```python
from build123d import *

# Parameters (mm, degrees)
BASE_SKETCH_W              = 127
BASE_SKETCH_H              = 147.5
BASE_SKETCH_R              = 5
BASE_DEPTH                 = 3
LEGS_SKETCH_W              = 5
LEGS_SKETCH_H              = 15
LEGS_DEPTH                 = 5
MOUNT_SKETCH_W             = 15
MOUNT_SKETCH_H             = 1
MOUNT_DEPTH                = 6
DONT_CUT_URSELF_R          = 6
MOUNTING_HOLE_SKETCH_R     = 1.5
MOUNTING_HOLE_1_DEPTH      = 2
MOUNTING_HOLE_2_SKETCH_R   = 1.5
MOUNTING_HOLE_2_DEPTH      = 2
MOUNT_2_SKETCH_W           = 15
MOUNT_2_SKETCH_H           = 1
MOUNT_2_DEPTH              = 6
DONT_CUT_URSELF_2_R        = 6
MOUNTING_HOLE_3_SKETCH_R   = 1.5
MOUNTING_HOLE_3_DEPTH      = 2
MOUNTING_HOLE_4_SKETCH_R   = 1.5
MOUNTING_HOLE_4_DEPTH      = 2
HOLES_FOR_PARTS_REACH      = 10
HOLES_FOR_PARTS_SKETCH_R   = 1.5
HOLES_FOR_PARTS_SKETCH_R_2 = 1.59


with BuildPart() as part:
    # Base Sketch → Base (new body)
    with BuildSketch(Plane(origin=(0, 0, 0), x_dir=(1, 0, 0), z_dir=(0, 1, 0))):
        Rectangle(BASE_SKETCH_W, BASE_SKETCH_H)
        Circle(BASE_SKETCH_R, mode=Mode.SUBTRACT)
    extrude(amount=BASE_DEPTH)

    # Legs Sketch → Legs (add)
    with BuildSketch(Plane.XZ):
        with Locations((-61, -66.25)):
            Rectangle(LEGS_SKETCH_W, LEGS_SKETCH_H)
        with Locations((61, -66.25)):
            Rectangle(LEGS_SKETCH_W, LEGS_SKETCH_H)
        with Locations((-61, 66.25)):
            Rectangle(LEGS_SKETCH_W, LEGS_SKETCH_H)
        with Locations((61, 66.25)):
            Rectangle(LEGS_SKETCH_W, LEGS_SKETCH_H)
    extrude(amount=LEGS_DEPTH)

    # Mount Sketch → Mount (add)
    with BuildSketch(Plane(origin=(63.5, 0, 0), x_dir=(0, 0, -1), z_dir=(1, 0, 0))):
        with Locations((-66.25, -4.5)):
            Rectangle(MOUNT_SKETCH_W, MOUNT_SKETCH_H)
        with Locations((66.25, -4.5)):
            Rectangle(MOUNT_SKETCH_W, MOUNT_SKETCH_H)
    extrude(amount=MOUNT_DEPTH)

    # Dont cut urself
    dont_cut_urself_edges = [part.edges().sort_by_distance(p)[0] for p in [
        (69.5, -4.5, 58.75),
        (69.5, -4.5, 73.75),
        (69.5, -4.5, -73.75),
        (69.5, -4.5, -58.75),
    ]]
    fillet(dont_cut_urself_edges, radius=DONT_CUT_URSELF_R)

    # Mounting Hole Sketch → Mounting Hole 1 (cut, through all)
    with BuildSketch(Plane(origin=(0, -4, 0), x_dir=(1, 0, 0), z_dir=(0, 1, 0))):
        with Locations((66.5, -66.25)):
            Circle(MOUNTING_HOLE_SKETCH_R)
    extrude(amount=-MOUNTING_HOLE_1_DEPTH, mode=Mode.SUBTRACT)

    # Mounting Hole 2 Sketch → Mounting Hole 2 (cut, through all)
    with BuildSketch(Plane(origin=(0, -4, 0), x_dir=(1, 0, 0), z_dir=(0, 1, 0))):
        with Locations((66.5, 66.25)):
            Circle(MOUNTING_HOLE_2_SKETCH_R)
    extrude(amount=-MOUNTING_HOLE_2_DEPTH, mode=Mode.SUBTRACT)

    # Mount 2 Sketch → Mount 2 (add)
    with BuildSketch(Plane.ZY.offset(63.5)):
        with Locations((-66.25, -4.5)):
            Rectangle(MOUNT_2_SKETCH_W, MOUNT_2_SKETCH_H)
        with Locations((66.25, -4.5)):
            Rectangle(MOUNT_2_SKETCH_W, MOUNT_2_SKETCH_H)
    extrude(amount=MOUNT_2_DEPTH)

    # Dont cut urself 2
    dont_cut_urself_2_edges = [part.edges().sort_by_distance(p)[0] for p in [
        (-69.5, -4.5, 73.75),
        (-69.5, -4.5, 58.75),
        (-69.5, -4.5, -58.75),
        (-69.5, -4.5, -73.75),
    ]]
    fillet(dont_cut_urself_2_edges, radius=DONT_CUT_URSELF_2_R)

    # Mounting Hole 3 Sketch → Mounting Hole 3 (cut, through all)
    with BuildSketch(Plane(origin=(0, -4, 0), x_dir=(1, 0, 0), z_dir=(0, 1, 0))):
        with Locations((-66.5, -66.25)):
            Circle(MOUNTING_HOLE_3_SKETCH_R)
    extrude(amount=-MOUNTING_HOLE_3_DEPTH, mode=Mode.SUBTRACT)

    # Mounting Hole 4 Sketch → Mounting Hole 4 (cut, through all)
    with BuildSketch(Plane(origin=(0, -4, 0), x_dir=(1, 0, 0), z_dir=(0, 1, 0))):
        with Locations((-66.5, 66.25)):
            Circle(MOUNTING_HOLE_4_SKETCH_R)
    extrude(amount=-MOUNTING_HOLE_4_DEPTH, mode=Mode.SUBTRACT)

    # Holes for Parts Sketch → Holes for Parts (cut, up to next)
    with BuildSketch(Plane(origin=(0, 3, 0), x_dir=(1, 0, 0), z_dir=(0, 1, 0)), mode=Mode.PRIVATE) as holes_for_parts_sk1:
        with Locations((31.75, -68.75)):
            Circle(HOLES_FOR_PARTS_SKETCH_R)
    holes_for_parts_tool1 = extrude(holes_for_parts_sk1.sketch, amount=-HOLES_FOR_PARTS_REACH, mode=Mode.PRIVATE) & part.part
    add(holes_for_parts_tool1.solids().sort_by_distance((31.75, 3, 68.75))[0], mode=Mode.SUBTRACT)
    # Holes for Parts Sketch → Holes for Parts (cut, up to next)
    with BuildSketch(Plane(origin=(0, 3, 0), x_dir=(1, 0, 0), z_dir=(0, 1, 0)), mode=Mode.PRIVATE) as holes_for_parts_sk2:
        with Locations((58.5, -53.875)):
            Circle(HOLES_FOR_PARTS_SKETCH_R)
    holes_for_parts_tool2 = extrude(holes_for_parts_sk2.sketch, amount=-HOLES_FOR_PARTS_REACH, mode=Mode.PRIVATE) & part.part
    add(holes_for_parts_tool2.solids().sort_by_distance((58.5, 3, 53.875))[0], mode=Mode.SUBTRACT)
    # Holes for Parts Sketch → Holes for Parts (cut, up to next)
    with BuildSketch(Plane(origin=(0, 3, 0), x_dir=(1, 0, 0), z_dir=(0, 1, 0)), mode=Mode.PRIVATE) as holes_for_parts_sk3:
        with Locations((5, -53.875)):
            Circle(HOLES_FOR_PARTS_SKETCH_R)
    holes_for_parts_tool3 = extrude(holes_for_parts_sk3.sketch, amount=-HOLES_FOR_PARTS_REACH, mode=Mode.PRIVATE) & part.part
    add(holes_for_parts_tool3.solids().sort_by_distance((5, 3, 53.875))[0], mode=Mode.SUBTRACT)
    # Holes for Parts Sketch → Holes for Parts (cut, up to next)
    with BuildSketch(Plane(origin=(0, 3, 0), x_dir=(1, 0, 0), z_dir=(0, 1, 0)), mode=Mode.PRIVATE) as holes_for_parts_sk4:
        with Locations((19.75, -15.25)):
            Circle(HOLES_FOR_PARTS_SKETCH_R)
    holes_for_parts_tool4 = extrude(holes_for_parts_sk4.sketch, amount=-HOLES_FOR_PARTS_REACH, mode=Mode.PRIVATE) & part.part
    add(holes_for_parts_tool4.solids().sort_by_distance((19.75, 3, 15.25))[0], mode=Mode.SUBTRACT)
    # Holes for Parts Sketch → Holes for Parts (cut, up to next)
    with BuildSketch(Plane(origin=(0, 3, 0), x_dir=(1, 0, 0), z_dir=(0, 1, 0)), mode=Mode.PRIVATE) as holes_for_parts_sk5:
        with Locations((-50.5, -16.25)):
            Circle(HOLES_FOR_PARTS_SKETCH_R)
    holes_for_parts_tool5 = extrude(holes_for_parts_sk5.sketch, amount=-HOLES_FOR_PARTS_REACH, mode=Mode.PRIVATE) & part.part
    add(holes_for_parts_tool5.solids().sort_by_distance((-50.5, 3, 16.25))[0], mode=Mode.SUBTRACT)
    # Holes for Parts Sketch → Holes for Parts (cut, up to next)
    with BuildSketch(Plane(origin=(0, 3, 0), x_dir=(1, 0, 0), z_dir=(0, 1, 0)), mode=Mode.PRIVATE) as holes_for_parts_sk6:
        with Locations((-24.5, -16.25)):
            Circle(HOLES_FOR_PARTS_SKETCH_R)
    holes_for_parts_tool6 = extrude(holes_for_parts_sk6.sketch, amount=-HOLES_FOR_PARTS_REACH, mode=Mode.PRIVATE) & part.part
    add(holes_for_parts_tool6.solids().sort_by_distance((-24.5, 3, 16.25))[0], mode=Mode.SUBTRACT)
    # Holes for Parts Sketch → Holes for Parts (cut, up to next)
    with BuildSketch(Plane(origin=(0, 3, 0), x_dir=(1, 0, 0), z_dir=(0, 1, 0)), mode=Mode.PRIVATE) as holes_for_parts_sk7:
        with Locations((-7.54, 33.19)):
            Circle(HOLES_FOR_PARTS_SKETCH_R_2)
    holes_for_parts_tool7 = extrude(holes_for_parts_sk7.sketch, amount=-HOLES_FOR_PARTS_REACH, mode=Mode.PRIVATE) & part.part
    add(holes_for_parts_tool7.solids().sort_by_distance((-7.54, 3, -33.19))[0], mode=Mode.SUBTRACT)
    # Holes for Parts Sketch → Holes for Parts (cut, up to next)
    with BuildSketch(Plane(origin=(0, 3, 0), x_dir=(1, 0, 0), z_dir=(0, 1, 0)), mode=Mode.PRIVATE) as holes_for_parts_sk8:
        with Locations((-7.54, 61.13)):
            Circle(HOLES_FOR_PARTS_SKETCH_R_2)
    holes_for_parts_tool8 = extrude(holes_for_parts_sk8.sketch, amount=-HOLES_FOR_PARTS_REACH, mode=Mode.PRIVATE) & part.part
    add(holes_for_parts_tool8.solids().sort_by_distance((-7.54, 3, -61.13))[0], mode=Mode.SUBTRACT)
    # Holes for Parts Sketch → Holes for Parts (cut, up to next)
    with BuildSketch(Plane(origin=(0, 3, 0), x_dir=(1, 0, 0), z_dir=(0, 1, 0)), mode=Mode.PRIVATE) as holes_for_parts_sk9:
        with Locations((44.53, 66.21)):
            Circle(HOLES_FOR_PARTS_SKETCH_R_2)
    holes_for_parts_tool9 = extrude(holes_for_parts_sk9.sketch, amount=-HOLES_FOR_PARTS_REACH, mode=Mode.PRIVATE) & part.part
    add(holes_for_parts_tool9.solids().sort_by_distance((44.53, 3, -66.21))[0], mode=Mode.SUBTRACT)
    # Holes for Parts Sketch → Holes for Parts (cut, up to next)
    with BuildSketch(Plane(origin=(0, 3, 0), x_dir=(1, 0, 0), z_dir=(0, 1, 0)), mode=Mode.PRIVATE) as holes_for_parts_sk10:
        with Locations((43.26, 17.95)):
            Circle(HOLES_FOR_PARTS_SKETCH_R_2)
    holes_for_parts_tool10 = extrude(holes_for_parts_sk10.sketch, amount=-HOLES_FOR_PARTS_REACH, mode=Mode.PRIVATE) & part.part
    add(holes_for_parts_tool10.solids().sort_by_distance((43.26, 3, -17.95))[0], mode=Mode.SUBTRACT)
    # Holes for Parts Sketch → Holes for Parts (cut, up to next)
    with BuildSketch(Plane(origin=(0, 3, 0), x_dir=(1, 0, 0), z_dir=(0, 1, 0)), mode=Mode.PRIVATE) as holes_for_parts_sk11:
        with Locations((50.5, -60.75)):
            Circle(HOLES_FOR_PARTS_SKETCH_R)
    holes_for_parts_tool11 = extrude(holes_for_parts_sk11.sketch, amount=-HOLES_FOR_PARTS_REACH, mode=Mode.PRIVATE) & part.part
    add(holes_for_parts_tool11.solids().sort_by_distance((50.5, 3, 60.75))[0], mode=Mode.SUBTRACT)
    # Holes for Parts Sketch → Holes for Parts (cut, up to next)
    with BuildSketch(Plane(origin=(0, 3, 0), x_dir=(1, 0, 0), z_dir=(0, 1, 0)), mode=Mode.PRIVATE) as holes_for_parts_sk12:
        with Locations((13, -60.75)):
            Circle(HOLES_FOR_PARTS_SKETCH_R)
    holes_for_parts_tool12 = extrude(holes_for_parts_sk12.sketch, amount=-HOLES_FOR_PARTS_REACH, mode=Mode.PRIVATE) & part.part
    add(holes_for_parts_tool12.solids().sort_by_distance((13, 3, 60.75))[0], mode=Mode.SUBTRACT)
    # Holes for Parts Sketch → Holes for Parts (cut, up to next)
    with BuildSketch(Plane(origin=(0, 3, 0), x_dir=(1, 0, 0), z_dir=(0, 1, 0)), mode=Mode.PRIVATE) as holes_for_parts_sk13:
        with Locations((13, -23.25)):
            Circle(HOLES_FOR_PARTS_SKETCH_R)
    holes_for_parts_tool13 = extrude(holes_for_parts_sk13.sketch, amount=-HOLES_FOR_PARTS_REACH, mode=Mode.PRIVATE) & part.part
    add(holes_for_parts_tool13.solids().sort_by_distance((13, 3, 23.25))[0], mode=Mode.SUBTRACT)
    # Holes for Parts Sketch → Holes for Parts (cut, up to next)
    with BuildSketch(Plane(origin=(0, 3, 0), x_dir=(1, 0, 0), z_dir=(0, 1, 0)), mode=Mode.PRIVATE) as holes_for_parts_sk14:
        with Locations((50.5, -23.25)):
            Circle(HOLES_FOR_PARTS_SKETCH_R)
    holes_for_parts_tool14 = extrude(holes_for_parts_sk14.sketch, amount=-HOLES_FOR_PARTS_REACH, mode=Mode.PRIVATE) & part.part
    add(holes_for_parts_tool14.solids().sort_by_distance((50.5, 3, 23.25))[0], mode=Mode.SUBTRACT)


solid = part.part
```
Source: CAD feature listing. Evaluate the final solid. Frame: model axes, mm. A direction names the side the tool comes from. Give positions to 0.01 mm unless a question says otherwise; leave off trailing zeros. Loops run counter-clockwise (first coordinate to the right, second up) from the corner with the lowest first, then second, coordinate; pieces in that order, holes last. Notation, with made-up numbers: M -28.75,29.5 L 22.25,29.5 A19 cw 22.25,53.5 Z; hole C 47.5,72 d8. An arc over 180 degrees is marked long. Put each result on its own line as item: value.
Q1. Mould query, pull axis X, two halves, no side actions, for faces 4 (the cylindrical face through (-1.08, 1.48, 4.88)), 5 (the cylindrical face through (-67.696, -4.493, -60.461)), 6 (the cylindrical face through (67.789, -4.493, -71.946)). Classes: released by +X, released by -X, zero draft, split by the parting line, or undercut.
Response values:
face 4: undercut
face 5: released by -X
face 6: released by +X
Q2. Pin query (flat end, axial travel): P1, Ø4, axis at x = 8, z = -10.5, coming from the -Y side; P2, Ø3.5, axis at x = -66.5, z = 66.25, coming from the -Y side; P3, Ø3, axis at x = 66.5, z = 66, coming from the +Y side. Return the tip coordinate at first contact, or that it passes through.
Response values:
P1: stops at y = 0
P2: stops at y = -5
P3: stops at y = -4
Q3. Line query: probe 1 along Z at (x, y) = (13, 2.25); probe 2 along X at (y, z) = (2.4, -17.95); probe 3 along Z at (x, y) = (0, 1.1). Output: solid intervals per line, ascending. Write a range as [from, to].
Response values:
probe 1: z = [-73.75, 21.75], [24.75, 59.25], [62.25, 73.75]
probe 2: x = [-63.5, 41.67], [44.85, 63.5]
probe 3: z = [-73.75, -5], [5, 73.75]
Q4. Section D-D (x = -40.5). Return the cut outline in (y, z), and give its area (4 significant figures).
Response values:
outline: M 0,-73.75 L 3,-73.75 L 3,73.75 L 0,73.75 Z
area: 442.5 mm²
Q5. Section B-B (x = 0). Return the cut outline in (y, z).
Response values:
outline: M 0,-73.75 L 3,-73.75 L 3,-5 L 0,-5 Z; M 0,5 L 3,5 L 3,73.75 L 0,73.75 Z
Q6. Section C-C (z = -41.5). Return the cut outline in (x, y), and give its area (3 significant figures).
Response values:
outline: M -63.5,0 L 63.5,0 L 63.5,3 L -63.5,3 Z
area: 381 mm²
Q7. Reachability of faces 1 (the flat face through (-63.5, 1, -1)), 2 (the flat face through (61, -3, 58.75)), 3 (the flat face through (-58.5, -2, 66)) from +Z, -Z, +X, -X, +Y, -Y: full face, straight path, thin tool, end or side. Return the list, or none.
Response values:
face 1: +Z, -Z, -X, +Y
face 2: +X, -X, -Y
face 3: +Z, -Z, -Y
Q8. Section A-A (y = -1.5). Return the cut outline in (x, z).
Response values:
outline: M -63.5,-73.75 L -58.5,-73.75 L -58.5,-58.75 L -63.5,-58.75 Z; M -63.5,58.75 L -58.5,58.75 L -58.5,73.75 L -63.5,73.75 Z; M 58.5,-73.75 L 63.5,-73.75 L 63.5,-58.75 L 58.5,-58.75 Z; M 58.5,58.75 L 63.5,58.75 L 63.5,73.75 L 58.5,73.75 Z
